from build123d import *

# Parameters (mm, degrees)
F0_R          = 5
F0_R_2        = 1.5
F1_DEPTH      = 3.5
F2_R          = 5
F2_R_2        = 4.25
F2_R_3        = 2.25
F2_R_4        = 1.5
F3_DEPTH      = 0.25
F3_DEPTH_BACK = 3.75
F4_SIZE       = 0.24999


# Not quite as in the source:
# - a fillet or chamfer is up to 0.001 mm smaller than in the source, because OpenCascade refuses the exact size


with BuildPart() as f1:
    # F0 (on Front) → F1 (new body)
    with BuildSketch(Plane.XZ):
        Circle(F0_R)
        Circle(F0_R_2, mode=Mode.SUBTRACT)
    extrude(amount=F1_DEPTH)

    # F2 (on face) → F3 (join, two sides)
    with BuildSketch(Plane.XZ.offset(3.5)) as f3_sk:
        Circle(F2_R)
        Circle(F2_R_2, mode=Mode.SUBTRACT)
        Circle(F2_R_3)
        Circle(F2_R_4, mode=Mode.SUBTRACT)
    extrude(amount=F3_DEPTH)
    extrude(f3_sk.sketch, amount=-F3_DEPTH_BACK)

    # F4 (size 0.25 in the source; OpenCascade refuses exactly that, so slightly less here)
    f4_edges = [f1.edges().sort_by_distance(p)[0] for p in [
        (-5, -3.75, 0),
        (-1.5, -3.75, 0),
        (-1.5, 0.25, 0),
        (-5, 0.25, 0),
    ]]
    chamfer(f4_edges, length=F4_SIZE)


solid = f1.part
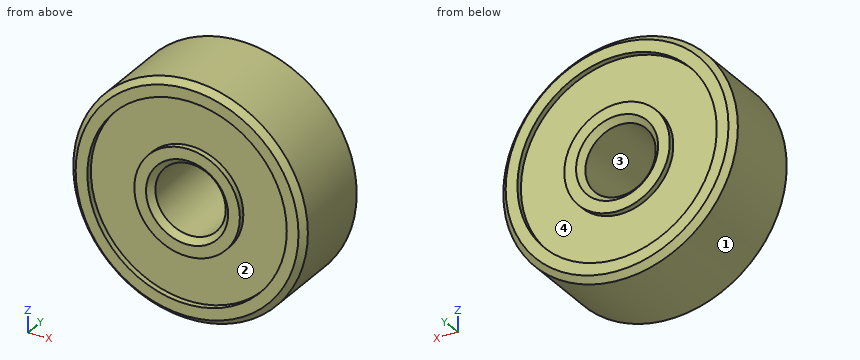
Design review of the part built by this model. Coordinates are the model's own, in mm. Face numbers are marked on the shaded views. A direction names the side the tool comes from. Coordinates: 2 decimals unless noted, no trailing zeros. Order: outer loops, then holes, each group sorted by start corner. A loop starts at its lowest first (then second) coordinate and runs counter-clockwise, first axis right, second up. Notation, with made-up numbers: (31, 12) - (75, 12) arc R18 ccw to (75, 17) - close; hole circle Ø4 at (-6, -3). An arc over 180 degrees is marked (long way). Put each result on its own line as item: value.
1) Take a section at C-C, the plane y = -2.05. Give the boundary of the cut face in (x, z).
Response values:
outline: circle Ø10 at (0, 0); hole circle Ø3 at (0, 0)
2) Tool access review of the marked faces 3 and 4: name each direction out of +Z, -Z, +X, -X, +Y, -Y from which nothing blocks a thin tool from reaching the whole face with its end or side.
Response values:
face 3: +Y, -Y
face 4: +Y
3) Wall thickness on L1, parallel to Z at x = 0, y = -2.3; L2, parallel to Z at x = 0, y = -3.65; L3, parallel to Z at x = 0, y = -3.6: over which ranges is each line inside the solid? List them lowest first. Write a range as from..to.
Response values:
L1: z = -5..-1.5, 1.5..5
L2: z = -4.85..-4.25, -2.25..-1.65, 1.65..2.25, 4.25..4.85
L3: z = -4.9..-4.25, -2.25..-1.6, 1.6..2.25, 4.25..4.9
4) The part is to be moulded in two halves that separate along Z. For the marked faces 1 and 2, say which applies: released by +Z, released by -Z, zero draft, split by the parting line, or undercut.
Response values:
face 1: split by the parting line
face 2: undercut
5) Insertion check: P1, Ø2, axis at y = -2.5, z = 2, coming from the +X side; P2, Ø2, axis at x = 1.5, y = -2, coming from the -Z side. Each pin has a flat end and moves straight along its axis. Give the tip position at first contact, or say it passes through.
Response values:
P1: stops at x = 4.9
P2: stops at z = -4.97
